```python
from build123d import *

# Parameters (mm, degrees)
SKETCH1_W                    = 47.3
SKETCH1_H                    = 42.3
BASE_FLANGE1_DEPTH           = 2.3
EDGE_FLANGE1_STRIP_W         = 13.2
EDGE_FLANGE1_STRIP_H         = 2.3
EDGE_FLANGE1_STRIP_CUT_DEPTH = 42.3
EDGE_FLANGE1_DEPTH           = 42.3
SKETCH9_W                    = 10.4
SKETCH9_H                    = 19
CUT_EXTRUDE1_DEPTH           = 3
SKETCH10_R                   = 1.5
CUT_EXTRUDE2_DEPTH           = 3
SKETCH11_R                   = 1.25
CUT_EXTRUDE5_DEPTH           = 3
SKETCH22_R                   = 6.95
CUT_EXTRUDE6_DEPTH           = 3


# Sheet-metal steps are written as plain solids
with BuildPart() as part:
    # Sketch1 → Base-Flange1 (new body)
    with BuildSketch(Plane.XY):
        with Locations((23.65, 21.15)):
            Rectangle(SKETCH1_W, SKETCH1_H)
    extrude(amount=-BASE_FLANGE1_DEPTH)

    # Edge-Flange1 strip (across the edge) → Edge-Flange1 strip cut (cut)
    with BuildSketch(Plane(origin=(47.3, 0, 0), x_dir=(-1, 0, 0), z_dir=(0, 1, 0))):
        with Locations((-2.3, -1.15)):
            Rectangle(EDGE_FLANGE1_STRIP_W, EDGE_FLANGE1_STRIP_H)
    extrude(amount=EDGE_FLANGE1_STRIP_CUT_DEPTH, mode=Mode.SUBTRACT)

    # Edge-Flange1 section (across the edge) → Edge-Flange1 (add)
    with BuildSketch(Plane(origin=(47.3, 0, 0), x_dir=(-1, 0, 0), z_dir=(0, 1, 0))):
        with BuildLine():
            Line((0, 2), (0, 23.7))
            Line((0, 23.7), (2.3, 23.7))
            Line((2.3, 23.7), (2.3, 2))
            ThreePointArc((2.3, 2), (2.885786438, 0.585786438), (4.3, 0))
            Line((4.3, 0), (4.3, -2.3))
            ThreePointArc((4.3, -2.3), (1.259440841, -1.040559159), (0, 2))
        make_face()
    extrude(amount=EDGE_FLANGE1_DEPTH)

    # Sketch9 → Cut-Extrude1 (cut)
    with BuildSketch(Plane(origin=(47.3, -232.998028616, -457.703147412), x_dir=(0, 0, -1), z_dir=(1, 0, 0))):
        with Locations((-472.38476551, 253.298028616)):
            Rectangle(SKETCH9_W, SKETCH9_H)
    extrude(amount=-CUT_EXTRUDE1_DEPTH, mode=Mode.SUBTRACT)

    # Sketch10 → Cut-Extrude2 (cut)
    with BuildSketch(Plane(origin=(47.3, -232.998028616, -457.703147412), x_dir=(0, 0, -1), z_dir=(1, 0, 0))):
        with Locations((-479.28476551, 268.298028616)):
            Circle(SKETCH10_R)
        with Locations((-462.68476551, 254.698028616)):
            Circle(SKETCH10_R)
        with Locations((-479.28476551, 238.298028616)):
            Circle(SKETCH10_R)
    extrude(amount=-CUT_EXTRUDE2_DEPTH, mode=Mode.SUBTRACT)

    # Sketch11 → Cut-Extrude5 (cut)
    with BuildSketch(Plane.XY):
        with Locations((5.65, 5.65)):
            Circle(SKETCH11_R)
        with Locations((5.65, 36.65)):
            Circle(SKETCH11_R)
        with Locations((36.65, 5.65)):
            Circle(SKETCH11_R)
        with Locations((36.65, 36.65)):
            Circle(SKETCH11_R)
    extrude(amount=-CUT_EXTRUDE5_DEPTH, mode=Mode.SUBTRACT)

    # Sketch22 → Cut-Extrude6 (cut)
    with BuildSketch(Plane.XY):
        with Locations((21.15, 21.15)):
            Circle(SKETCH22_R)
    extrude(amount=-CUT_EXTRUDE6_DEPTH, mode=Mode.SUBTRACT)


solid = part.part
```
Build history of the part. All positions in model axes, mm. A direction names the side the tool comes from. Give positions to 0.01 mm unless a question says otherwise; leave off trailing zeros. Order: outer loops, then holes, each group sorted by start corner. A loop starts at its lowest first (then second) coordinate and runs counter-clockwise, first axis right, second up. Notation, with made-up numbers: M 82,37.25 L 112,37.25 A9 ccw 112,45.25 Z; hole C 66,76 d9. An arc over 180 degrees is marked long. Return JSON: item names as keys, results as strings.
Q1. Wall check: probe 1 along Y at (x, z) = (5.65, -0.85); probe 2 along X at (y, z) = (4, 18.5); probe 3 along Z at (x, y) = (15.5, 12). Give the ranges that are in metal, low to high. Write a range as from..to.
Answer list:
{"probe 1": "y = 0..4.4, 6.9..35.4, 37.9..42.3", "probe 2": "x = 45..47.3", "probe 3": "z = -2.3..0"}
Q2. Two-plate mould, pull along Z, no slides. Class faces 4 (the face through (4.729, 6.495, -1.134)), 5 (the face through (46.166, 23.187, 5.177)), 6 (the face through (21, 12, 0)), 7 (the face through (46.01, 20.85, -1.07)): pulls with the +Z half, pulls with the -Z half, needs draft (parallel to the pull), parting line crosses it, or undercut.
Answer list:
{"face 4": "needs draft", "face 5": "undercut", "face 6": "pulls with the +Z half", "face 7": "pulls with the -Z half"}
Q3. Band-saw the part on C-C (y = 31). Give the cut face in (x, z).
Answer list:
{"outline": "M 0,-2.3 L 43,-2.3 A4.3 ccw 47.3,2 L 47.3,23.7 L 45,23.7 L 45,2 A2 cw 43,0 L 0,0 Z"}
Q4. Band-saw the part on B-B (x = 25.5). Give the cut face in (y, z), then the cut area to 3 significant figures.
Answer list:
{"outline": "M 0,-2.3 L 15.73,-2.3 L 15.73,0 L 0,0 Z; M 26.57,-2.3 L 42.3,-2.3 L 42.3,0 L 26.57,0 Z", "area": "72.4 mm^2"}
Q5. Flat gauge pins, fed straight in: pin 1 (2 mm diameter, centred on x = 36.65, y = 36.65, fed in from +Z); pin 2 (1.8 mm diameter, centred on x = 46.5, y = 24.5, fed in from -Z); pin 3 (5 mm diameter, centred on y = 34, z = 16.5, fed in from -X); pin 4 (2 mm diameter, centred on x = 42, y = 32.5, fed in from +Z). Where does each tip first touch, or does it go through?
Answer list:
{"pin 1": "passes through", "pin 2": "stops at z = -1.42", "pin 3": "stops at x = 45", "pin 4": "stops at z = 0"}
Q6. 3-axis set-ups, long thin cutter, end or side, ignore diameter. For faces 1 (the face through (46, 29.8, 15)), 2 (the face through (46, 21, 23.7)), 3 (the face through (45, 21, 8)): which of +Z, -Z, +X, -X, +Y, -Y reach the whole face in a straight line?
Answer list:
{"face 1": "+X, -X", "face 2": "+Z, +X, -X, +Y, -Y", "face 3": "+Z, -X, +Y, -Y"}
Q7. Band-saw the part on D-D (y = 15). Give the cut face in (x, z), then the cut area to 3 significant figures.
Answer list:
{"outline": "M 0,-2.3 L 17.91,-2.3 L 17.91,0 L 0,0 Z; M 24.39,-2.3 L 43,-2.3 A4.3 ccw 47.3,2 L 47.3,9.48 L 45,9.48 L 45,2 A2 cw 43,0 L 24.39,0 Z; M 45,19.88 L 47.3,19.88 L 47.3,23.7 L 45,23.7 Z", "area": "121 mm^2"}
Q8. Band-saw the part on A-A (z = 13.5). Give the cut face in (x, y), then the cut area to 3 significant figures.
Answer list:
{"outline": "M 45,0 L 47.3,0 L 47.3,10.8 L 45,10.8 Z; M 45,29.8 L 47.3,29.8 L 47.3,42.3 L 45,42.3 Z", "area": "53.6 mm^2"}
